The figure shows three views and two pictorial views of one solid part (mm, origin at its lowest corner). Answer the questions. A direction names the side the tool comes from. Coordinates: 2 decimals unless noted, no trailing zeros. Write each loop counter-clockwise with the first axis right and the second up, starting at its lowest first coordinate (ties: lowest second). Pieces come first, ordered by that corner, then holes. Notation, with made-up numbers: M -22.5,10 L 18.5,10 A17 ccw 18.5,35 Z; hole C -25.5,11.5 d3. An arc over 180 degrees is marked long. Use a Markdown table: item, result. Add a question column.
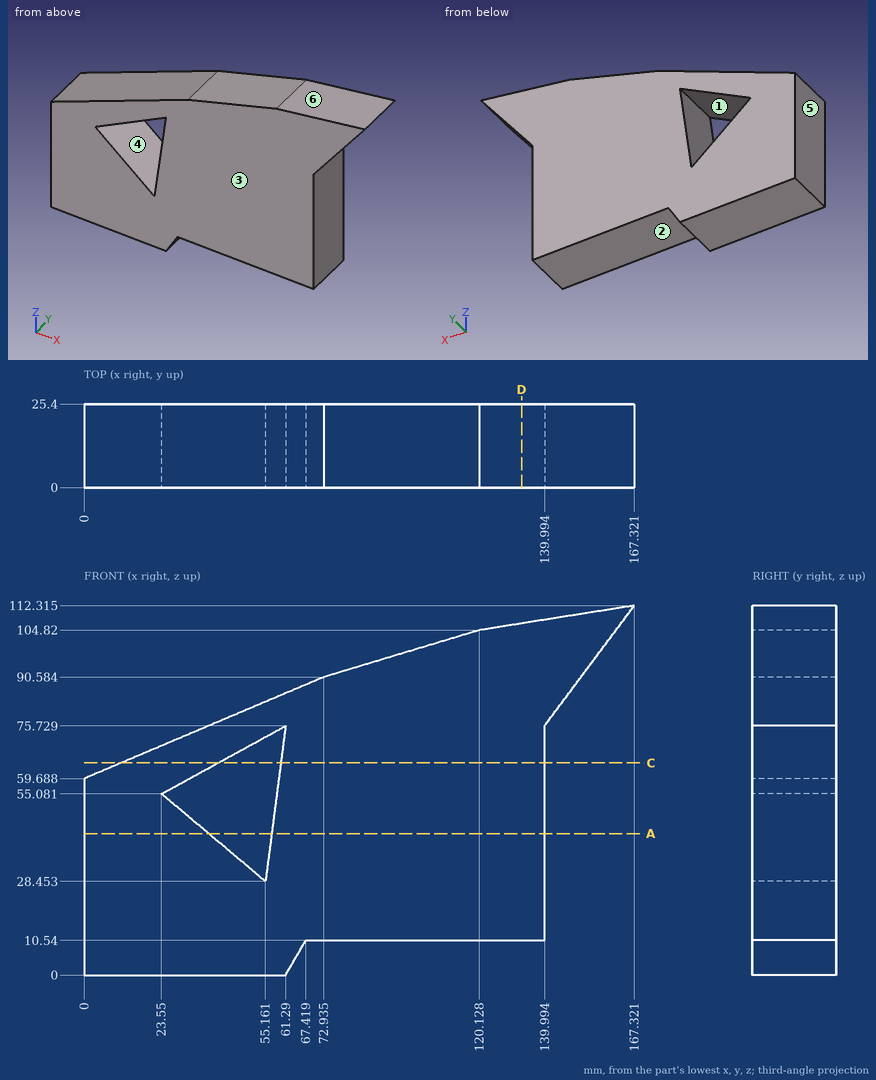
Item 1: For the marked faces 1, 2 and 3, determine the directions among +Z, -Z, +X, -X, +Y, -Y from which every point of the face is accessible in a straight line to the end or side of a thin tool.
Item 2: Determine the mould class of the marked faces 4, 5 and 6 for opening direction Z: pulls with the +Z half, pulls with the -Z half, needs draft (parallel to the pull), parting line crosses it, or undercut.
Item 3: Consider probe 1 along X at (y, z) = (9.75, 64.5) (1 decimal); probe 2 along X at (y, z) = (18.5, 27); probe 3 along X at (y, z) = (11.25, 44) (1 decimal). Determine where each line is inside the solid, lowest interval first.
Item 4: Find section A-A on z = 43. Give the vertices of the cut face in (x, y).
Item 5: Find section D-D on x = 133. Give the vertices of the cut face in (y, z) (1 decimal), then the cut area to 3 significant figures.
Item 6: Find section C-C on z = 64.5. Give the vertices of the cut face in (x, y) (1 decimal).
Item 7: Each of these flat-tipped pins is pushed along its axis until it touches: pin 1 (1 mm diameter, centred on x = 82.5, y = 8, fed in from +Z); pin 2 (2 mm diameter, centred on x = 88, y = 18.5, fed in from -Z); pin 3 (5 mm diameter, centred on x = 144, y = 14.5, fed in from -Z) (1 decimal). Where does it stop, or does it pass through?
Geometry says:
| question | item | result |
|---|---|---|
| 1 | face 1 | +Y, -Y |
| 1 | face 2 | -Z, +X, +Y, -Y |
| 1 | face 3 | +Z, -Z, +X, -X, -Y |
| 2 | face 4 | undercut |
| 2 | face 5 | needs draft |
| 2 | face 6 | pulls with the +Z half |
| 3 | probe 1 | x = 11.4 to 40.8, 59.8 to 140 |
| 3 | probe 2 | x = 0 to 139.99 |
| 3 | probe 3 | x = 0 to 36.7, 57.2 to 140 |
| 4 | outline | M 0,0 L 37.89,0 L 37.89,25.4 L 0,25.4 Z; M 57.05,0 L 139.99,0 L 139.99,25.4 L 57.05,25.4 Z |
| 5 | outline | M 0,10.5 L 25.4,10.5 L 25.4,106.9 L 0,106.9 Z |
| 5 | area | 2,450 mm2 |
| 6 | outline | M 11.4,0 L 40.8,0 L 40.8,25.4 L 11.4,25.4 Z; M 59.8,0 L 140,0 L 140,25.4 L 59.8,25.4 Z |
| 7 | pin 1 | stops at z = 93.62 |
| 7 | pin 2 | stops at z = 10.54 |
| 7 | pin 3 | stops at z = 77.7 |
